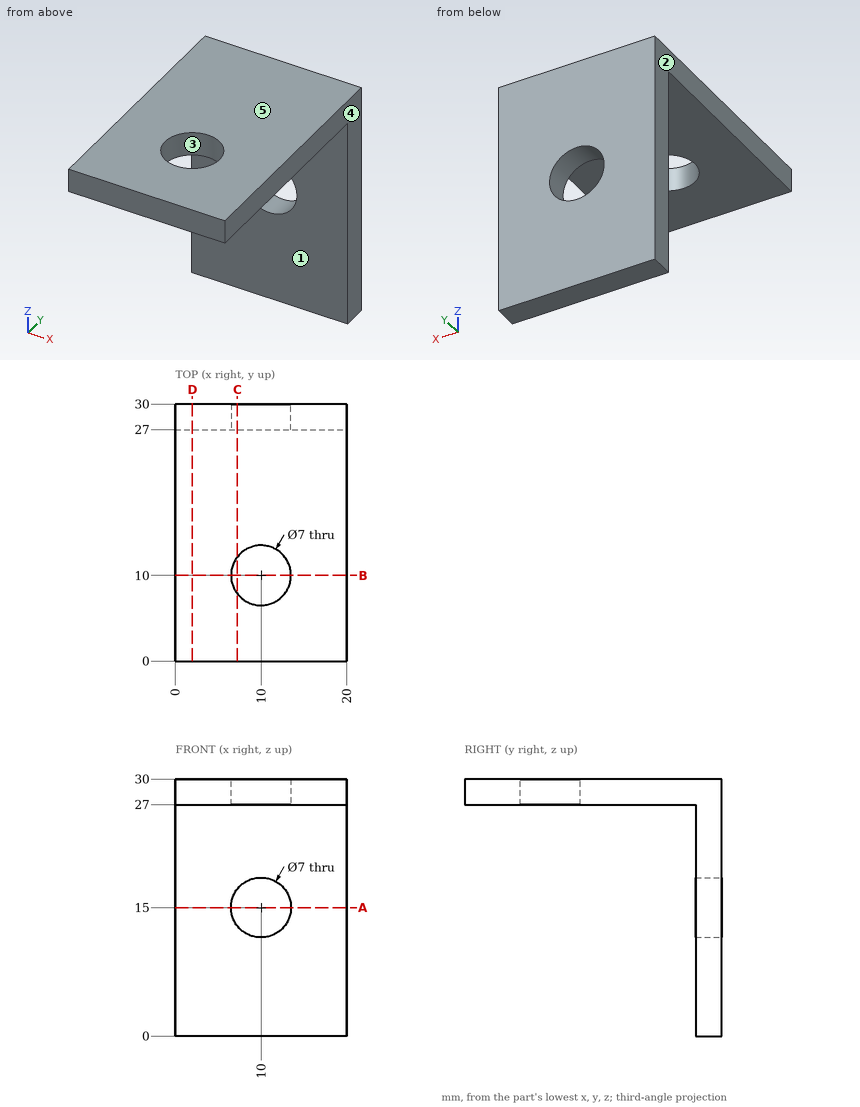
Part print with two shaded views. Sizes in mm from the minimum x, y, z corner. A direction names the side the tool comes from. Round coordinates to 2 decimals unless told otherwise and drop trailing zeros. Loops run counter-clockwise (first coordinate to the right, second up) from the corner with the lowest first, then second, coordinate; pieces in that order, holes last. Notation, with made-up numbers: M -20.5,37.25 L 34.5,37.25 A34 ccw 34.5,68.25 Z; hole C 57,36.5 d5. An arc over 180 degrees is marked long. Put each result on its own line as item: value. Start each with the question number.
Item 1: Mould opens along X. For the marked faces 3, 4 and 5 say: released by +X, released by -X, zero draft, split by the parting line, or undercut.
Item 2: Drill centre lines: line 1 along Y through (x, z) = (10, 27.7); line 2 along Z through (x, y) = (10, 29); line 3 along Y through (x, z) = (6.5, 6.5). Where is each one in solid material? Low to high.
Item 3: Cut at D-D (x = 2). List the corners of the cut face in (y, z).
Item 4: Cut at C-C (x = 7.25). List the corners of the cut face in (y, z).
Item 5: 3-axis set-ups, long thin cutter, end or side, ignore diameter. For the marked faces 1 and 2: which of +Z, -Z, +X, -X, +Y, -Y reach the whole face in a straight line?
Item 6: Cut at A-A (z = 15). List the corners of the cut face in (x, y).
Item 7: Drop flat-ended pins along their axis: P1, Ø6, axis at x = 5.5, z = 10.5, coming from the -Y side; P2, Ø10, axis at x = 10.5, y = 20, coming from the -Z side. Give the stop position or say it passes through.
Answer block:
1. face 3: undercut
1. face 4: released by +X
1. face 5: zero draft
2. line 1: 0 to 6.5, 13.5 to 30
2. line 2: 0 to 11.5, 18.5 to 30
2. line 3: 27 to 30
3. outline: M 0,27 L 27,27 L 27,0 L 30,0 L 30,30 L 0,30 Z
4. outline: M 0,27 L 7.83,27 L 7.83,30 L 0,30 Z; M 12.17,27 L 27,27 L 27,17.17 L 30,17.17 L 30,30 L 12.17,30 Z; M 27,0 L 30,0 L 30,12.83 L 27,12.83 Z
5. face 1: -Z, +X, -X, -Y
5. face 2: +Z, -Z, -X, +Y, -Y
6. outline: M 0,27 L 6.5,27 L 6.5,30 L 0,30 Z; M 13.5,27 L 20,27 L 20,30 L 13.5,30 Z
7. P1: y = 27
7. P2: z = 27
